Verification items for this drawing (mm, ordinates from the low corner). Coordinates: 2 decimals unless noted, no trailing zeros. Loops run counter-clockwise (first coordinate to the right, second up) from the corner with the lowest first, then second, coordinate; pieces in that order, holes last.
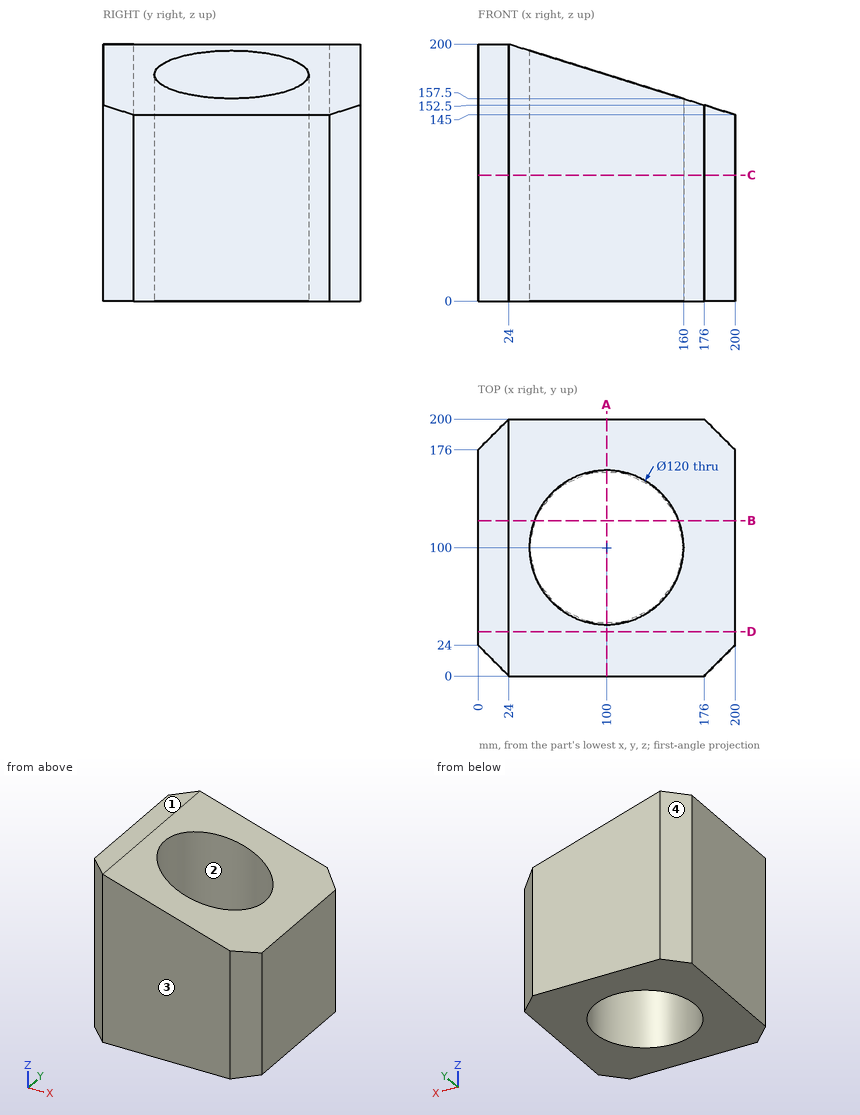
(1) Section check C-C, the plane z = 98. Enter the section's corners in (x, y), plus the area to 3 significant figures.
(2) Section check D-D, the plane y = 34.5. Enter the section's corners in (x, z), plus the area to 3 significant figures.
(3) Section check A-A, the plane x = 100. Enter the section's corners in (y, z).
(4) Gauge pin test, flat end, axial feed: P1, Ø12, axis at x = 168.5, y = 154.5, coming from the +Z side. Record the tip position at first contact, or that the pin passes through.
(5) Draft check along Y on the marked faces 1, 2, 3 and 4. Enter one of: pulls with the +Y half, pulls with the -Y half, needs draft (parallel to the pull), parting line crosses it, or undercut.
(6) Section check B-B, the plane y = 121. Enter the section's corners in (x, z).
(7) Scan lines: line 1 along Y through (x, z) = (100, 57.5); line 2 along Z through (x, y) = (40, 156); line 3 along X through (y, z) = (119, 122.5). Record each from-to range of solid material in increasing order.
Determined:
1. outline: (0, 24) - (24, 0) - (176, 0) - (200, 24) - (200, 176) - (176, 200) - (24, 200) - (0, 176) - close; hole circle Ø120 at (100, 100)
1. area: 27,500 mm2
2. outline: (0, 0) - (200, 0) - (200, 145) - (24, 200) - (0, 200) - close
2. area: 35,200 mm2
3. outline: (0, 0) - (40, 0) - (40, 176.25) - (0, 176.25) - close; (160, 0) - (200, 0) - (200, 176.25) - (160, 176.25) - close
4. P1: stops at z = 156.72
5. face 1: needs draft
5. face 2: undercut
5. face 3: pulls with the -Y half
5. face 4: pulls with the +Y half
6. outline: (0, 0) - (43.8, 0) - (43.8, 193.81) - (24, 200) - (0, 200) - close; (156.2, 0) - (200, 0) - (200, 145) - (156.2, 158.69) - close
7. line 1: y = 0 to 40, 160 to 200
7. line 2: z = 0 to 195
7. line 3: x = 0 to 43.09, 156.91 to 200
